Build history of the part. All positions in model axes, mm. Face numbers are marked on the shaded views. Coordinates: 2 decimals unless noted, no trailing zeros. Order: outer loops, then holes, each group sorted by start corner. A loop starts at its lowest first (then second) coordinate and runs counter-clockwise, first axis right, second up. Notation, with made-up numbers: (46.5, 57.25) - (63.5, 57.25) arc R15 ccw to (63.5, 76.25) - close; hole circle Ø1 at (82, 70). An arc over 180 degrees is marked (long way). Write each question's results on one line, items separated by ' | '.
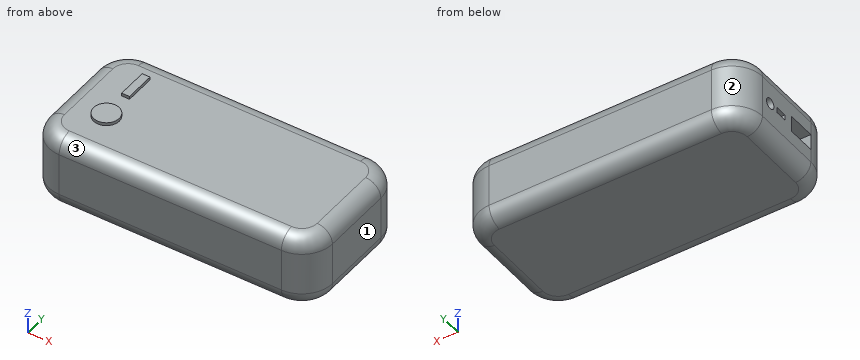
from build123d import *

# Parameters (mm, degrees)
CROQUIS1_W              = 93
CROQUIS1_H              = 43.6
SALIENTE_EXTRUIR1_DEPTH = 24
REDONDEO1_R             = 10
REDONDEO2_R             = 5
CROQUIS2_R              = 1.795301333
CROQUIS2_W              = 5.26615661
CROQUIS2_H              = 9.314898328
CROQUIS2_W_2            = 1.780690374
CROQUIS2_H_2            = 3.893669573
CORTAR_EXTRUIR1_DEPTH   = 10
CROQUIS4_R              = 4.202442578
CROQUIS4_W              = 2.57850106
CROQUIS4_H              = 9.991691608
SALIENTE_EXTRUIR2_DEPTH = 1


with BuildPart() as part:
    # Croquis1 → Saliente-Extruir1 (new body)
    with BuildSketch(Plane.XY):
        Rectangle(CROQUIS1_W, CROQUIS1_H)
    extrude(amount=SALIENTE_EXTRUIR1_DEPTH)

    # Redondeo1
    redondeo1_edges = [part.edges().sort_by_distance(p)[0] for p in [
        (46.5, -21.8, 12),
        (-46.5, -21.8, 12),
        (-46.5, 21.8, 12),
        (46.5, 21.8, 12),
    ]]
    fillet(redondeo1_edges, radius=REDONDEO1_R)

    # Redondeo2
    redondeo2_edges = [part.edges().sort_by_distance(p)[0] for p in [
        (46.5, 0, 0),
        (46.5, 0, 24),
        (0, -21.8, 0),
        (-46.5, 0, 0),
        (0, 21.8, 0),
        (-43.571067812, 18.871067812, 0),
        (-43.571067812, -18.871067812, 0),
        (43.571067812, 18.871067812, 0),
        (43.571067812, -18.871067812, 0),
        (0, -21.8, 24),
        (0, 21.8, 24),
        (-46.5, 0, 24),
        (-43.571067812, 18.871067812, 24),
        (-43.571067812, -18.871067812, 24),
        (43.571067812, 18.871067812, 24),
        (43.571067812, -18.871067812, 24),
    ]]
    fillet(redondeo2_edges, radius=REDONDEO2_R)

    # Croquis2 → Cortar-Extruir1 (cut)
    with BuildSketch(Plane.ZY.offset(46.5)):
        with Locations((12, 7.984643734)):
            Circle(CROQUIS2_R)
        with Locations((12, -7.142550836)):
            Rectangle(CROQUIS2_W, CROQUIS2_H)
        with Locations((12, 2.792227185)):
            Rectangle(CROQUIS2_W_2, CROQUIS2_H_2)
    extrude(amount=-CORTAR_EXTRUIR1_DEPTH, mode=Mode.SUBTRACT)

    # Croquis4 → Saliente-Extruir2 (add)
    with BuildSketch(Plane.XY.offset(24)):
        with Locations((-31.747794301, -5.801627385)):
            Circle(CROQUIS4_R)
        with Locations((-31.747794301, 8.541284761)):
            Rectangle(CROQUIS4_W, CROQUIS4_H)
    extrude(amount=SALIENTE_EXTRUIR2_DEPTH)


solid = part.part
1. Band-saw the part on B-B on z = 12. Give the cut face in (x, y), then the cut area to 3 significant figures.
Solved:
outline: (-46.5, -11.8) arc R10 ccw to (-36.5, -21.8) - (36.5, -21.8) arc R10 ccw to (46.5, -11.8) - (46.5, 11.8) arc R10 ccw to (36.5, 21.8) - (-36.5, 21.8) arc R10 ccw to (-46.5, 11.8) - (-46.5, 9.78) - (-36.5, 9.78) - (-36.5, 6.19) - (-46.5, 6.19) - (-46.5, 4.74) - (-36.5, 4.74) - (-36.5, 0.85) - (-46.5, 0.85) - (-46.5, -2.49) - (-36.5, -2.49) - (-36.5, -11.8) - close | area: 3,800 mm2
2. Band-saw the part on C-C on z = 6.25. Give the cut face in (x, y).
Solved:
outline: (-46.5, -11.8) arc R10 ccw to (-36.5, -21.8) - (36.5, -21.8) arc R10 ccw to (46.5, -11.8) - (46.5, 11.8) arc R10 ccw to (36.5, 21.8) - (-36.5, 21.8) arc R10 ccw to (-46.5, 11.8) - close
3. Two-plate mould, pull along Y, no slides. Class the marked faces 1, 2 and 3: +Y half, -Y half, draft (parallel to the pull), parting line (faces both ways), or undercut.
Solved:
face 1: draft | face 2: +Y half | face 3: -Y half
4. Drop flat-ended pins along their axis: pin 1 Ø0.5 at (x, z) = (-41, 12) entering from +Y; pin 2 Ø7.5 at (x, y) = (-43.5, -7) entering from +Z; pin 3 Ø1.6 at (x, z) = (-42.5, 13) entering from +Y; pin 4 Ø2 at (x, z) = (37, 6.5) entering from -Y. Give the stop position or say it passes through.
Solved:
pin 1: stops at y = 20.85 | pin 2: stops at z = 24 | pin 3: stops at y = 20.34 | pin 4: stops at y = -21.8
5. Band-saw the part on A-A on x = 19. Give the cut face in (y, z), then the cut area to 3 significant figures.
Solved:
outline: (-21.8, 5) arc R5 ccw to (-16.8, 0) - (16.8, 0) arc R5 ccw to (21.8, 5) - (21.8, 19) arc R5 ccw to (16.8, 24) - (-16.8, 24) arc R5 ccw to (-21.8, 19) - close | area: 1,020 mm2
6. Probe line 1 (Y direction, x = -41, z = 12); line 2 (Y direction, x = -39, z = 12); line 3 (Z direction, x = 7.5, y = -16). List the from-to ranges inside material, lowest first.
Solved:
line 1: y = -20.73 to -11.8, -2.49 to 0.85, 4.74 to 6.19, 9.78 to 20.73 | line 2: y = -21.48 to -11.8, -2.49 to 0.85, 4.74 to 6.19, 9.78 to 21.48 | line 3: z = 0 to 24
